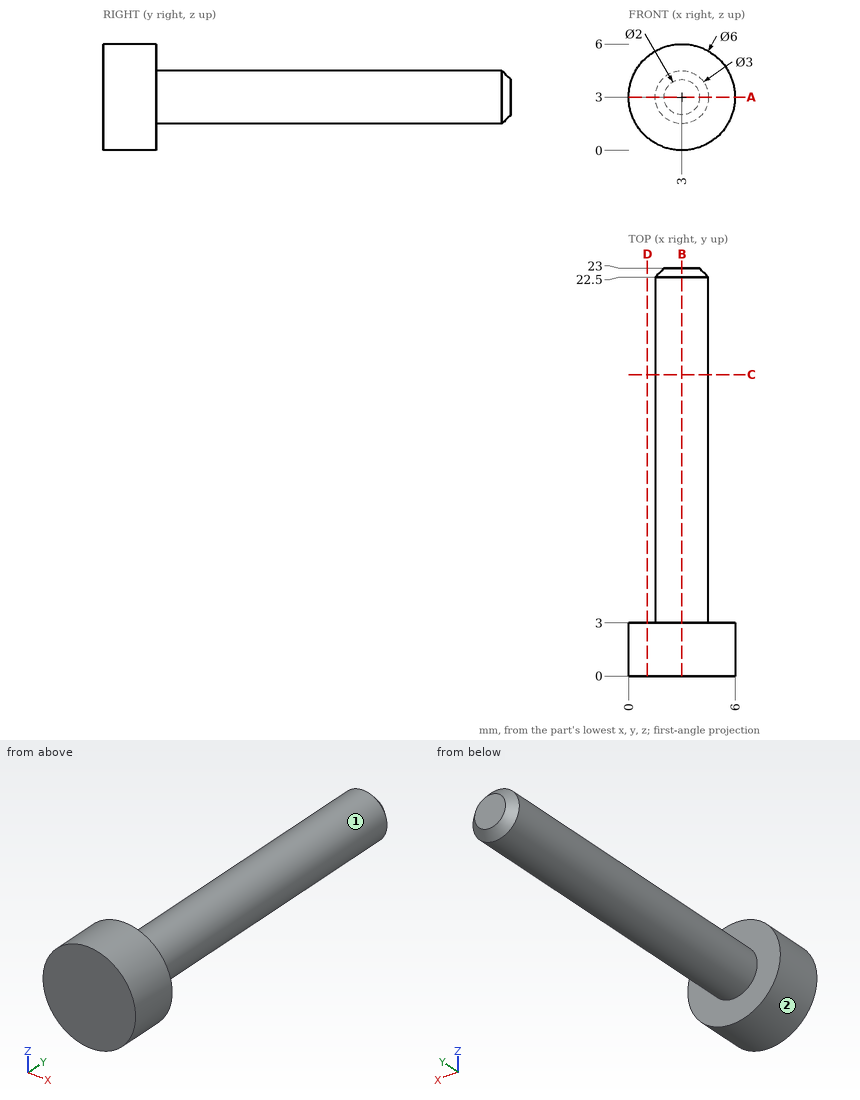
Geometry check sheet. Reference: drawing and pictorial views, mm from the part's lowest x, y, z. A direction names the side the tool comes from. Coordinates: 2 decimals unless noted, no trailing zeros. Write each loop counter-clockwise with the first axis right and the second up, starting at its lowest first coordinate (ties: lowest second). Pieces come first, ordered by that corner, then holes.
Item 1: Scan lines: probe 1 along Y at (x, z) = (4.6, 4.9); probe 2 along X at (y, z) = (12, 2.95); probe 3 along Z at (x, y) = (2.85, 21). Record each from-to range of solid material in increasing order.
Numbers:
probe 1: y = 0 to 3
probe 2: x = 1.5 to 4.5
probe 3: z = 1.51 to 4.49
Item 2: Access from +Z, -Z, +X, -X, +Y, -Y to the whole of each face (thin tool, end or side, straight path). Record for the marked faces 1 and 2.
Numbers:
face 1: +Y
face 2: +Y, -Y
Item 3: Cross-section at A-A on z = 3. Record the boundary of the cut face in (x, y).
Numbers:
outline: (0, 0) - (6, 0) - (6, 3) - (4.5, 3) - (4.5, 22.5) - (4, 23) - (2, 23) - (1.5, 22.5) - (1.5, 3) - (0, 3) - close
Item 4: Cross-section at C-C on y = 17. Record the boundary of the cut face in (x, z), then the cut area to 3 significant figures.
Numbers:
outline: circle Ø3 at (3, 3)
area: 7.07 mm2
Item 5: Cross-section at B-B on x = 3. Record the boundary of the cut face in (y, z).
Numbers:
outline: (0, 0) - (3, 0) - (3, 1.5) - (22.5, 1.5) - (23, 2) - (23, 4) - (22.5, 4.5) - (3, 4.5) - (3, 6) - (0, 6) - close
Item 6: Cross-section at D-D on x = 1.05. Record the boundary of the cut face in (y, z).
Numbers:
outline: (0, 0.72) - (3, 0.72) - (3, 5.28) - (0, 5.28) - close
Item 7: Depth check by flat-ended pin: pin 1 Ø2 at (x, z) = (3.5, 5) entering from -Y; pin 2 Ø1.5 at (x, y) = (4.5, 11.5) entering from -Z; pin 3 Ø3 at (x, y) = (4.5, 9) entering from -Z; pin 4 Ø1.5 at (x, y) = (1, 20) entering from -Z. Enter the tip coordinate at first touch or a pass-through.
Numbers:
pin 1: stops at y = 0
pin 2: stops at z = 1.7
pin 3: stops at z = 1.5
pin 4: stops at z = 2.17
